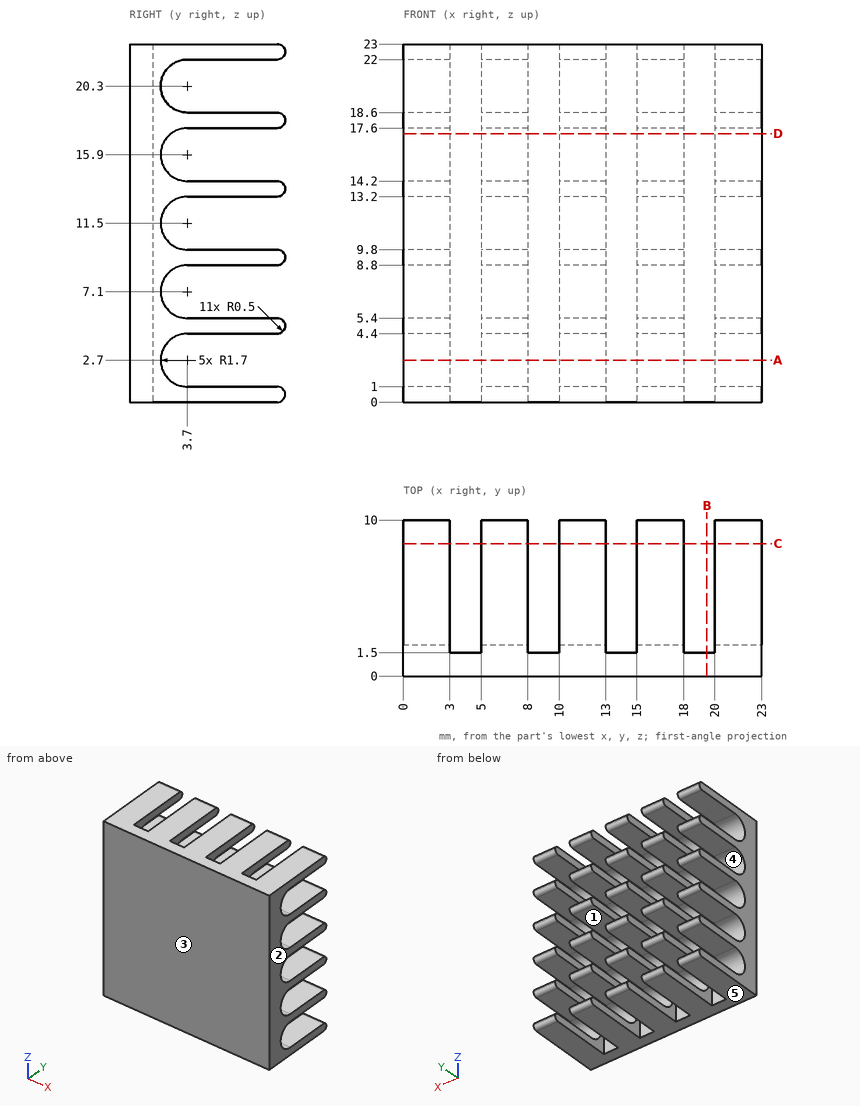
Could you check a few things on this drawing? It's one solid part, dimensions in mm from its lowest x, y, z. A direction names the side the tool comes from. Give positions to 0.01 mm unless a question says otherwise; leave off trailing zeros. Write each loop counter-clockwise with the first axis right and the second up, starting at its lowest first coordinate (ties: lowest second). Pieces come first, ordered by that corner, then holes.
(1) Will these pins go through, and if not, where does the flat tip stop? pin 1 (2.5 mm diameter, centred on x = 16.5, y = 5.5, fed in from -Z); pin 2 (1.6 mm diameter, centred on x = 13.5, z = 14.5, fed in from +Y).
Output values:
pin 1: stops at z = 0
pin 2: stops at y = 9.97
(2) If I drill on L1, parallel to Z at x = 5.75, y = 4.5; L2, parallel to X at y = 3, z = 13.5; L3, parallel to Y at x = 13.5, z = 17.5, over which ranges is the centre line in solid material (lowest first)?
Output values:
L1: z = 0 to 1, 4.4 to 5.4, 8.8 to 9.8, 13.2 to 14.2, 17.6 to 18.6, 22 to 23
L2: x = 0 to 3, 5 to 8, 10 to 13, 15 to 18, 20 to 23
L3: y = 0 to 1.5
(3) Imagine slicing it at A-A, the plane z = 2.7. Write out the boundary of the cut face in (x, y), and give its area (3 significant figures).
Output values:
outline: (0, 0) - (23, 0) - (23, 2) - (20, 2) - (20, 1.5) - (18, 1.5) - (18, 2) - (15, 2) - (15, 1.5) - (13, 1.5) - (13, 2) - (10, 2) - (10, 1.5) - (8, 1.5) - (8, 2) - (5, 2) - (5, 1.5) - (3, 1.5) - (3, 2) - (0, 2) - close
area: 42.0 mm2
(4) Thinking about a two-plate mould opening in Z: for the marked faces 3, 4 and 5, which applies, pulls with the +Z half, pulls with the -Z half, needs draft (parallel to the pull), parting line crosses it, or undercut?
Output values:
face 3: needs draft
face 4: undercut
face 5: pulls with the -Z half
(5) Imagine slicing it at B-B, the plane x = 19.5. Write out the boundary of the cut face in (y, z), and give its area (3 significant figures).
Output values:
outline: (0, 0) - (1.5, 0) - (1.5, 23) - (0, 23) - close
area: 34.5 mm2
(6) Imagine slicing it at D-D, the plane z = 17.25. Write out the boundary of the cut face in (x, y).
Output values:
outline: (0, 0) - (23, 0) - (23, 2.67) - (20, 2.67) - (20, 1.5) - (18, 1.5) - (18, 2.67) - (15, 2.67) - (15, 1.5) - (13, 1.5) - (13, 2.67) - (10, 2.67) - (10, 1.5) - (8, 1.5) - (8, 2.67) - (5, 2.67) - (5, 1.5) - (3, 1.5) - (3, 2.67) - (0, 2.67) - close
(7) On a 3-axis mill with a long thin cutter (end or side, diameter ignored), from which of +Z, -Z, +X, -X, +Y, -Y can I reach the whole of each face in a straight line? I mean the marked faces 1 and 2. Say none if no direction works.
Output values:
face 1: +X, -X, +Y
face 2: +Z, -Z, +X, +Y, -Y
(8) Imagine slicing it at C-C, the plane y = 8.5. Count the separate pieces of the cut face and the enclosed holes in it, and give its area (3 significant figures).
Output values:
separate pieces: 30
enclosed holes: 0
area: 90.0 mm2
